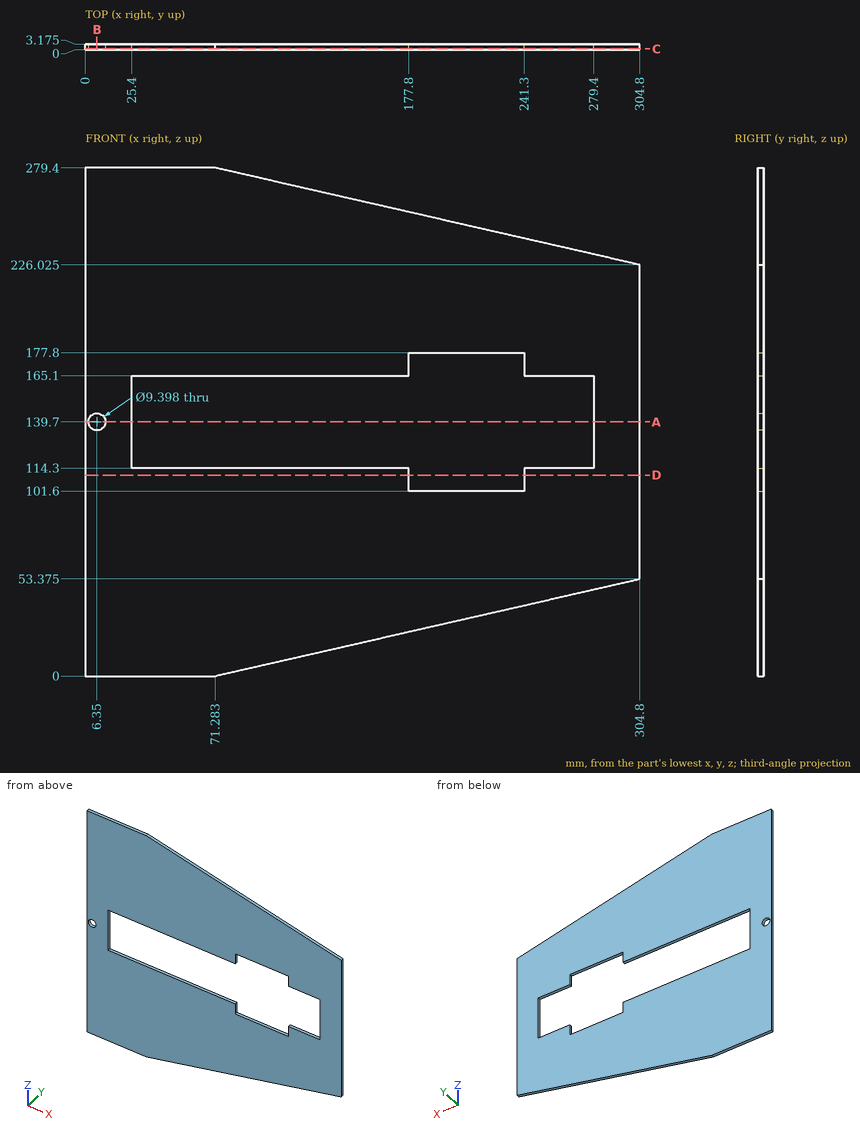
Job drawing, mm, ordinate dimensions from the low corner. One solid piece. Coordinates: 2 decimals unless noted, no trailing zeros. Write each loop counter-clockwise with the first axis right and the second up, starting at its lowest first coordinate (ties: lowest second). Pieces come first, ordered by that corner, then holes.
Item 1: Slice it at A-A (z = 139.7). Write the cut outline in (x, y) (1 decimal).
Item 2: Pin check, flat tips, straight feed: pin 1 (1 mm diameter, centred on x = 124.5, y = 1.5, fed in from +Z); pin 2 (1 mm diameter, centred on x = 223, y = 2.5, fed in from +Z); pin 3 (1.6 mm diameter, centred on x = 263, y = 2, fed in from -Z). Stop position of each tip, or through.
Item 3: Probe line 1 (X direction, y = 2.1, z = 139.7); line 2 (Z direction, x = 61, y = 0.5); line 3 (X direction, y = 2.65, z = 119.5). List the from-to ranges inside material, lowest first.
Item 4: Slice it at C-C (y = 0.5). Count the separate pieces of the cut face and the enclosed holes in it, and give its area (3 significant figures).
Item 5: Slice it at B-B (x = 6.35). Write the cut outline in (y, z) (1 decimal).
Item 6: Slice it at D-D (z = 110.5). Write the cut outline in (x, y) (1 decimal), and give its area (3 significant figures).
Results found:
1. outline: (0, 0) - (1.7, 0) - (1.7, 3.2) - (0, 3.2) - close; (11, 0) - (25.4, 0) - (25.4, 3.2) - (11, 3.2) - close; (279.4, 0) - (304.8, 0) - (304.8, 3.2) - (279.4, 3.2) - close
2. pin 1: stops at z = 267.35
2. pin 2: stops at z = 244.84
2. pin 3: stops at z = 43.64
3. line 1: x = 0 to 1.65, 11.05 to 25.4, 279.4 to 304.8
3. line 2: z = 0 to 114.3, 165.1 to 279.4
3. line 3: x = 0 to 25.4, 279.4 to 304.8
4. separate pieces: 1
4. enclosed holes: 2
4. area: 58,100 mm2
5. outline: (0, 0) - (3.2, 0) - (3.2, 135) - (0, 135) - close; (0, 144.4) - (3.2, 144.4) - (3.2, 279.4) - (0, 279.4) - close
6. outline: (0, 0) - (177.8, 0) - (177.8, 3.2) - (0, 3.2) - close; (241.3, 0) - (304.8, 0) - (304.8, 3.2) - (241.3, 3.2) - close
6. area: 766 mm2
